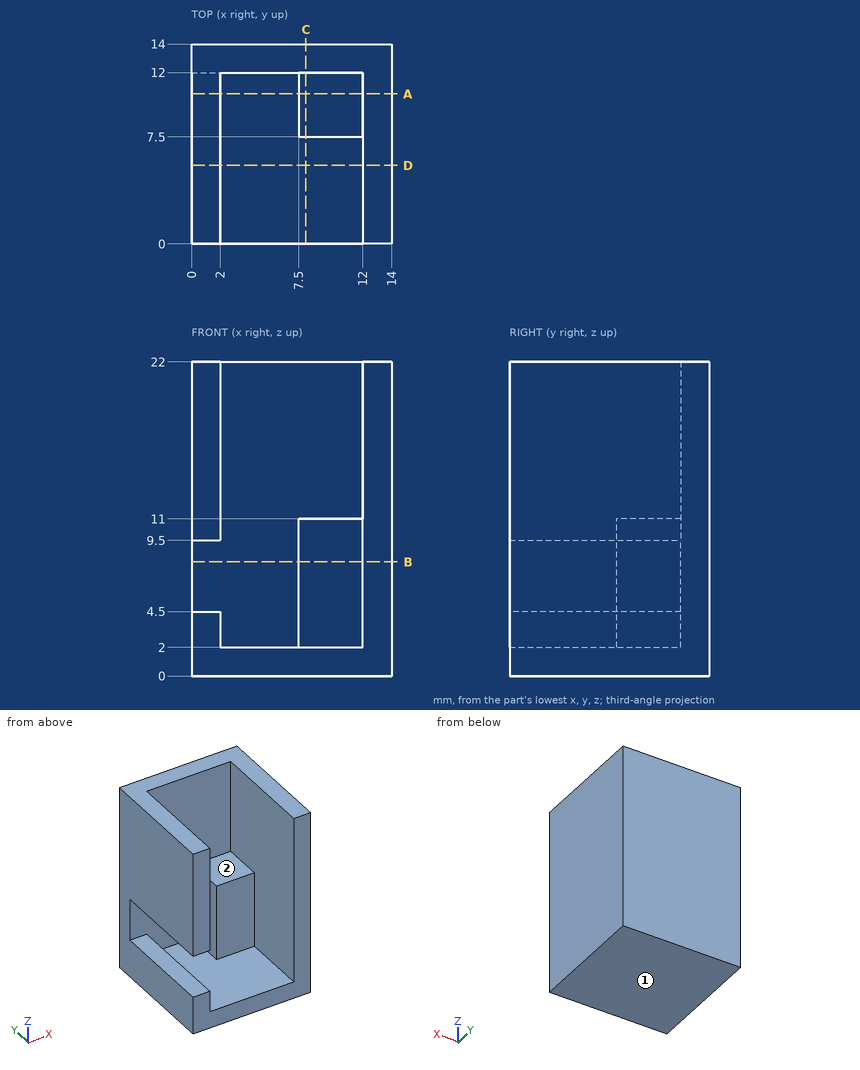
For this review, use the dimensioned drawing (mm, ordinates from the lowest corner) and the shaded views. A direction names the side the tool comes from. Round coordinates to 2 decimals unless told otherwise and drop trailing zeros. Order: outer loops, then holes, each group sorted by start corner. A loop starts at its lowest first (then second) coordinate and runs counter-clockwise, first axis right, second up. Notation, with made-up numbers: M 40.5,-23 L 81.5,-23 A16 ccw 81.5,1 Z; hole C 1.25,27 d5. An arc over 180 degrees is marked long. Use a Markdown table: item, result. Add a question column.
Item 1: Add section D-D, the plane y = 5.5. Give the boundary of the cut face in (x, z), then the cut area to 3 significant figures.
Item 2: Add section A-A, the plane y = 10.5. Give the boundary of the cut face in (x, z), then the cut area to 4 significant figures.
Item 3: Add section C-C, the plane x = 8. Give the boundary of the cut face in (y, z), then the cut area to 4 significant figures.
Item 4: Tool access review of the marked faces 1 and 2: name each direction out of +Z, -Z, +X, -X, +Y, -Y from which nothing blocks a thin tool from reaching the whole face with its end or side.
Item 5: Add section B-B, the plane z = 8. Give the boundary of the cut face in (x, y), then the cut area to 4 significant figures.
Item 6: Insertion check: pin 1 (5 mm diameter, centred on x = 7, y = 9, fed in from +Z); pin 2 (3 mm diameter, centred on x = 5, y = 8.5, fed in from +Z). Each pin has a flat end and moves straight along its axis. Give the tip position at first contact, or say it passes through.
Item 7: To check wall thickness, follow line 1 along X through (y, z) = (7.5, 14.75); line 2 along Z through (x, y) = (1.5, 4.5); line 3 along Z through (x, y) = (9.75, 6.5). State the ranges of each line that lie inside material, in increasing order.
Geometry results:
| question | item | result |
|---|---|---|
| 1 | outline | M 0,0 L 14,0 L 14,22 L 12,22 L 12,2 L 2,2 L 2,4.5 L 0,4.5 Z; M 0,9.5 L 2,9.5 L 2,22 L 0,22 Z |
| 1 | area | 98.0 mm² |
| 2 | outline | M 0,0 L 14,0 L 14,22 L 12,22 L 12,11 L 7.5,11 L 7.5,2 L 2,2 L 2,4.5 L 0,4.5 Z; M 0,9.5 L 2,9.5 L 2,22 L 0,22 Z |
| 2 | area | 138.5 mm² |
| 3 | outline | M 0,0 L 14,0 L 14,22 L 12,22 L 12,11 L 7.5,11 L 7.5,2 L 0,2 Z |
| 3 | area | 108.5 mm² |
| 4 | face 1 | -Z, +X, -X, +Y, -Y |
| 4 | face 2 | +Z, -Y |
| 5 | outline | M 0,12 L 7.5,12 L 7.5,7.5 L 12,7.5 L 12,0 L 14,0 L 14,14 L 0,14 Z |
| 5 | area | 72.25 mm² |
| 6 | pin 1 | stops at z = 11 |
| 6 | pin 2 | stops at z = 2 |
| 7 | line 1 | x = 0 to 2, 12 to 14 |
| 7 | line 2 | z = 0 to 4.5, 9.5 to 22 |
| 7 | line 3 | z = 0 to 2 |
